Print and shaded views of the part. All mm, measured from the part's lowest x, y and z. Round coordinates to 2 decimals unless told otherwise and drop trailing zeros. Write each loop counter-clockwise with the first axis right and the second up, starting at its lowest first coordinate (ties: lowest second). Pieces come first, ordered by that corner, then holes. Notation, with made-up numbers: (42.25, -32) -> (52.25, -32) arc R16 ccw to (52.25, -22) -> close; hole circle Ø4 at (-17.75, -19.5). An arc over 180 degrees is marked (long way). Use CSV: the item, a comma, the result in double quotes. Start each with the question number.
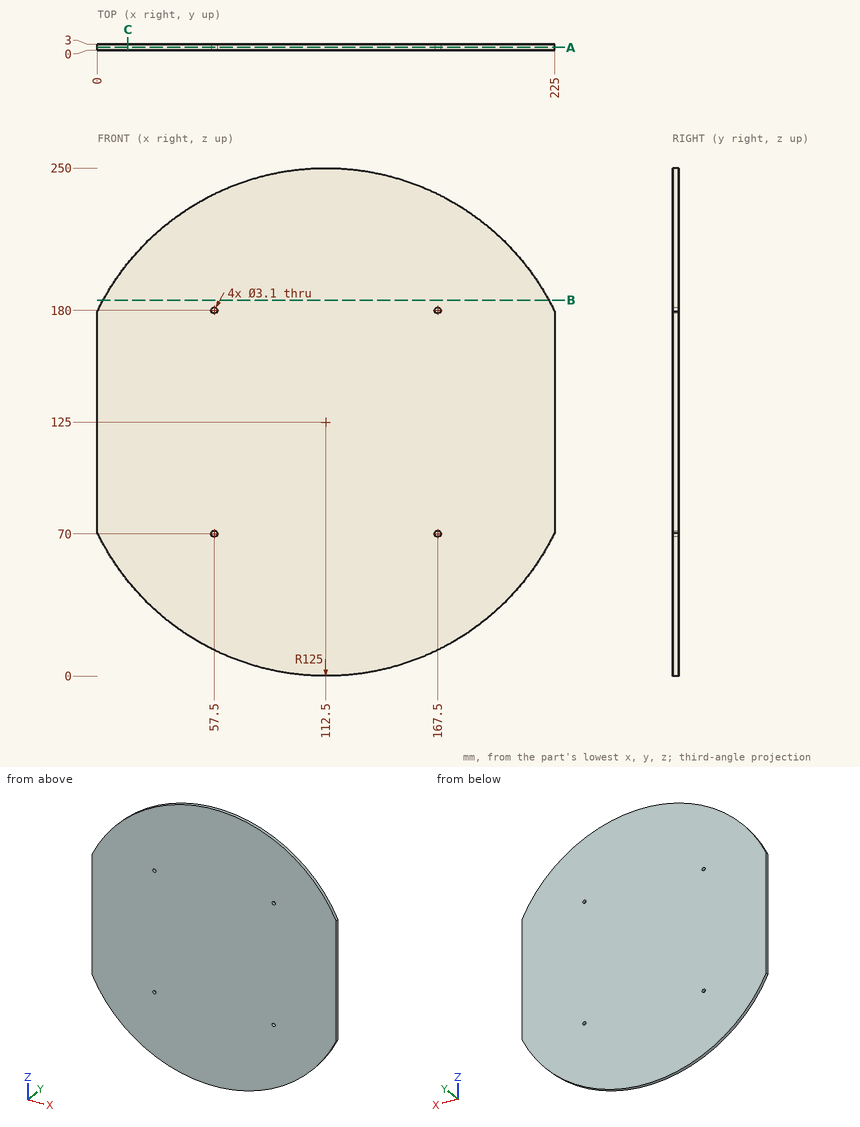
1. Band-saw the part on A-A (y = 1.3). List the corners of the cut face in (x, z).
2. Drill centre lines: line 1 along Z through (x, y) = (167, 0.3); line 2 along X through (y, z) = (1.2, 70); line 3 along Z through (x, y) = (167.5, 0.7). Where is each one in solid material? Low to high. Write a range as [from, to].
3. Band-saw the part on B-B (z = 185). List the corners of the cut face in (x, y), then the cut area to 3 significant figures.
4. Flat gauge pins, fed straight in: pin 1 (1.5 mm diameter, centred on x = 159.5, y = 1, fed in from -Z); pin 2 (3 mm diameter, centred on x = 57.5, z = 180, fed in from +Y); pin 3 (1 mm diameter, centred on x = 137.5, y = 1.5, fed in from -Z); pin 4 (1.5 mm diameter, centred on x = 66.5, y = 1, fed in from -Z). Where does each tip first touch, or does it go through?
5. Band-saw the part on C-C (x = 15). List the corners of the cut face in (y, z), then the cut area to 3 significant figures.
Answers below:
1,outline,"(0, 70.51) arc R125 ccw to (225, 70.51) -> (225, 179.49) arc R125 ccw to (0, 179.49) -> close; hole circle Ø3.1 at (57.5, 70); hole circle Ø3.1 at (57.5, 180); hole circle Ø3.1 at (167.5, 70); hole circle Ø3.1 at (167.5, 180)"
2,line 1,"z = [12.51, 68.53], [71.47, 178.53], [181.47, 237.49]"
2,line 2,"x = [0.25, 55.95], [59.05, 165.95], [169.05, 224.75]"
2,line 3,"z = [12.75, 68.45], [71.55, 178.45], [181.55, 237.25]"
3,outline,"(2.84, 0) -> (222.16, 0) -> (222.16, 3) -> (2.84, 3) -> close"
3,area,"658 mm^2"
4,pin 1,"stops at z = 8.87"
4,pin 2,"passes through"
4,pin 3,"stops at z = 2.42"
4,pin 4,"stops at z = 8.48"
5,outline,"(0, 46.78) -> (3, 46.78) -> (3, 203.22) -> (0, 203.22) -> close"
5,area,"469 mm^2"
